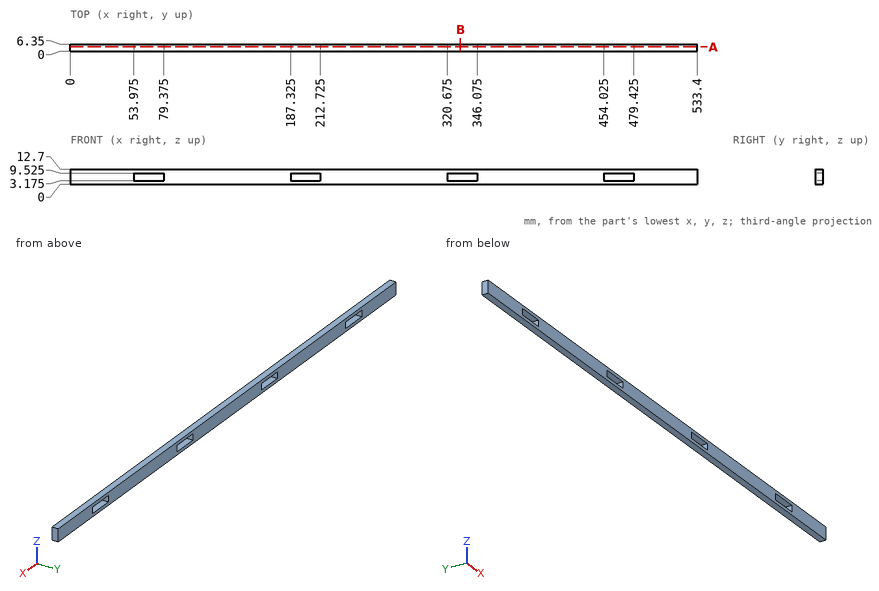
Print and shaded views of the part. All mm, measured from the part's lowest x, y and z. Round coordinates to 2 decimals unless told otherwise and drop trailing zeros. Write each loop counter-clockwise with the first axis right and the second up, starting at its lowest first coordinate (ties: lowest second). Pieces come first, ordered by that corner, then holes. Notation, with made-up numbers: (65.25, 54) -> (69.25, 54) arc R17 ccw to (69.25, 85) -> close; hole circle Ø5 at (-35, 31.25). An arc over 180 degrees is marked (long way). Answer in a Markdown table with one row per item. Add a question column.
Item 1: Drop a flat-ended pin along its axis: pin 1 Ø4 at (x, z) = (266.5, 3) entering from -Y. Give the stop position or say it passes through.
Item 2: Drill centre lines: line 1 (X direction, y = 5.25, z = 6) (3 decimals); line 2 (Z direction, x = 62.5, y = 2.5) (3 decimals). Where is each one in solid material? Low to high. Write a range as from..to.
Item 3: Saw through at A-A, the plane y = 4. Write the cut outline in (x, z) (3 decimals), then the cut area to 3 significant figures.
Item 4: Saw through at B-B, the plane x = 332. Write the cut outline in (y, z) (3 decimals), then the cut area to 3 significant figures.
Findings below:
| question | item | result |
|---|---|---|
| 1 | pin 1 | stops at y = 0 |
| 2 | line 1 | x = 0..53.975, 79.375..187.325, 212.725..320.675, 346.075..454.025, 479.425..533.4 |
| 2 | line 2 | z = 0..3.175, 9.525..12.7 |
| 3 | outline | (0, 0) -> (533.4, 0) -> (533.4, 12.7) -> (0, 12.7) -> close; hole (53.975, 3.175) -> (79.375, 3.175) -> (79.375, 9.525) -> (53.975, 9.525) -> close; hole (187.325, 3.175) -> (212.725, 3.175) -> (212.725, 9.525) -> (187.325, 9.525) -> close; hole (320.675, 3.175) -> (346.075, 3.175) -> (346.075, 9.525) -> (320.675, 9.525) -> close; hole (454.025, 3.175) -> (479.425, 3.175) -> (479.425, 9.525) -> (454.025, 9.525) -> close |
| 3 | area | 6,130 mm^2 |
| 4 | outline | (0, 0) -> (6.35, 0) -> (6.35, 3.175) -> (0, 3.175) -> close; (0, 9.525) -> (6.35, 9.525) -> (6.35, 12.7) -> (0, 12.7) -> close |
| 4 | area | 40.3 mm^2 |
